from build123d import *

# Parameters (mm, degrees)
F0_R     = 14.2875
F1_DEPTH = 25.4
F2_DEPTH = 50.8


with BuildPart() as f1:
    # F0 (on Front) → F1 (new body)
    with BuildSketch(Plane.XZ):
        with BuildLine():
            ThreePointArc((4.7625, -28.17533), (21.824517, -18.445083), (28.575, 0))
            ThreePointArc((28.575, 0), (21.824517, 18.445083), (4.7625, 28.17533))
            ThreePointArc((4.7625, 28.17533), (-28.575, 0), (4.7625, -28.17533))
        make_face()
        with BuildLine():
            ThreePointArc((-13.470384, 4.7625), (0, 14.2875), (13.470384, 4.7625))
            Line((13.470384, 4.7625), (19.05, 4.7625))
            Line((19.05, 4.7625), (19.05, -4.7625))
            Line((19.05, -4.7625), (13.470384, -4.7625))
            ThreePointArc((13.470384, -4.7625), (0, -14.2875), (-13.470384, -4.7625))
            Line((-13.470384, -4.7625), (-19.05, -4.7625))
            Line((-19.05, -4.7625), (-19.05, 4.7625))
            Line((-19.05, 4.7625), (-13.470384, 4.7625))
        make_face(mode=Mode.SUBTRACT)
        with BuildLine():
            ThreePointArc((4.7625, 28.17533), (21.824517, 18.445083), (28.575, 0))
            ThreePointArc((28.575, 0), (21.824517, -18.445083), (4.7625, -28.17533))
            Line((4.7625, -28.17533), (60.325, -18.783553))
            ThreePointArc((60.325, -18.783553), (38.1, 0), (60.325, 18.783553))
            Line((60.325, 18.783553), (4.7625, 28.17533))
        make_face()
        with BuildLine():
            ThreePointArc((76.2, 0), (71.699678, 12.296722), (60.325, 18.783553))
            ThreePointArc((60.325, 18.783553), (38.1, 0), (60.325, -18.783553))
            ThreePointArc((60.325, -18.783553), (71.699678, -12.296722), (76.2, 0))
        make_face()
        with Locations((57.15, 0)):
            Circle(F0_R, mode=Mode.SUBTRACT)
        with BuildLine():
            ThreePointArc((-13.470384, -4.7625), (-14.2875, 0), (-13.470384, 4.7625))
            Line((-13.470384, 4.7625), (-19.05, 4.7625))
            Line((-19.05, 4.7625), (-19.05, -4.7625))
            Line((-19.05, -4.7625), (-13.470384, -4.7625))
        make_face()
    extrude(amount=F1_DEPTH)

    # F0 (on Front) → F2 (join)
    with BuildSketch(Plane.XZ):
        with BuildLine():
            ThreePointArc((4.7625, -28.17533), (21.824517, -18.445083), (28.575, 0))
            ThreePointArc((28.575, 0), (21.824517, 18.445083), (4.7625, 28.17533))
            ThreePointArc((4.7625, 28.17533), (-28.575, 0), (4.7625, -28.17533))
        make_face()
        with BuildLine():
            ThreePointArc((-13.470384, 4.7625), (0, 14.2875), (13.470384, 4.7625))
            Line((13.470384, 4.7625), (19.05, 4.7625))
            Line((19.05, 4.7625), (19.05, -4.7625))
            Line((19.05, -4.7625), (13.470384, -4.7625))
            ThreePointArc((13.470384, -4.7625), (0, -14.2875), (-13.470384, -4.7625))
            Line((-13.470384, -4.7625), (-19.05, -4.7625))
            Line((-19.05, -4.7625), (-19.05, 4.7625))
            Line((-19.05, 4.7625), (-13.470384, 4.7625))
        make_face(mode=Mode.SUBTRACT)
        with BuildLine():
            ThreePointArc((-13.470384, -4.7625), (-14.2875, 0), (-13.470384, 4.7625))
            Line((-13.470384, 4.7625), (-19.05, 4.7625))
            Line((-19.05, 4.7625), (-19.05, -4.7625))
            Line((-19.05, -4.7625), (-13.470384, -4.7625))
        make_face()
    extrude(amount=F2_DEPTH)


solid = f1.part
Here's how the part is built. I have some questions about the finished solid (model axes, mm). A direction names the side the tool comes from. Coordinates: 2 decimals unless noted, no trailing zeros. Write each loop counter-clockwise with the first axis right and the second up, starting at its lowest first coordinate (ties: lowest second). Pieces come first, ordered by that corner, then holes.
Item 1: If I drill on line 1 (X direction, y = -5, z = -11); line 2 (X direction, y = -5.5, z = 13); line 3 (Y direction, x = 39.5, z = 3.5), over which ranges is the centre line in solid material (lowest first)?
Item 2: If we mould it in two halves opening along Z, with no side actions, what happens to faces 3 (the flat face through (23, 0, 0)), 4 (the flat face through (32.155, -12.522, -23.545)), 5 (the flat face through (32.933, -12.522, 23.414)), 6 (the flat face through (19.05, -25, 0))? For each: +Z half, -Z half, draft (parallel to the pull), parting line (faces both ways), or undercut.
Item 3: I want a section at C-C on z = -12. Write out the boundary of the cut face in (x, y), and give its area (3 significant figures).
Item 4: On a 3-axis mill with a long thin cutter (end or side, diameter ignored), from which of +Z, -Z, +X, -X, +Y, -Y can I reach the whole of each face in a straight line? I mean faces 1 (the flat face through (16, -25, -4.762)), 2 (the flat face through (-13, -50.8, 7)). Say none if no direction works.
Item 5: I want a section at B-B on x = 0. Write out the boundary of the cut face in (y, z) (1 decimal), and give its area (3 significant figures).
Item 6: I want a section at D-D on y = -13.5. Count the separate pieces of the cut face and the enclosed holes in it, and give its area (3 significant figures).
Item 7: Will these pins go through, and if not, where does the flat tip stop? pin 1 (6 mm diameter, centred on x = -14.5, y = -9.5, fed in from +Z); pin 2 (2 mm diameter, centred on x = 29, z = 0, fed in from +Y); pin 3 (1 mm diameter, centred on y = -14, z = -11, fed in from -X); pin 4 (4 mm diameter, centred on y = -39, z = 4.5, fed in from +X).
Findings below:
1. line 1: x = -26.37 to -9.12, 9.12 to 48.03, 66.27 to 72.7
1. line 2: x = -25.45 to -5.93, 5.93 to 51.22, 63.08 to 71.07
1. line 3: y = -25.4 to 0
2. face 3: draft
2. face 4: -Z half
2. face 5: +Z half
2. face 6: undercut
3. outline: (-25.93, -50.8) - (-7.75, -50.8) - (-7.75, 0) - (-25.93, 0) - close; (7.75, -50.8) - (25.93, -50.8) - (25.93, -25.4) - (49.4, -25.4) - (49.4, 0) - (7.75, 0) - close; (64.9, -25.4) - (71.95, -25.4) - (71.95, 0) - (64.9, 0) - close
3. area: 2,620 mm2
4. face 1: +Y, -Y
4. face 2: +Z, -Z, +X, -X, -Y
5. outline: (-50.8, -28.6) - (0, -28.6) - (0, -14.3) - (-50.8, -14.3) - close; (-50.8, 14.3) - (0, 14.3) - (0, 28.6) - (-50.8, 28.6) - close
5. area: 1,450 mm2
6. separate pieces: 1
6. enclosed holes: 2
6. area: 3,280 mm2
7. pin 1: stops at z = 26.16
7. pin 2: stops at y = 0
7. pin 3: stops at x = -26.58
7. pin 4: stops at x = 28.47
